Geometry: see drawing. Coordinates: mm, zero at the bounding-box minimum. A direction names the side the tool comes from. Round coordinates to 2 decimals unless told otherwise and drop trailing zeros. Loops run counter-clockwise (first coordinate to the right, second up) from the corner with the lowest first, then second, coordinate; pieces in that order, holes last.
(1) First-contact query: pin 1 Ø1 at (y, z) = (7.5, 36) entering from -X; pin 2 Ø3.5 at (y, z) = (13, 21.8) entering from -X; pin 3 Ø5 at (x, y) = (14, 2) entering from +Z. Flat tips, straight axial feed; report the tip coordinate or a pass-through.
(2) Cut plane C-C, the plane y = 12.25. Output: boundary loops of the cut face in (x, z), and give its area (3 significant figures).
(3) Draft query along Y for the marked faces 1, 2 and 3. Return one class per face: released by +Y, released by -Y, zero draft, split by the parting line, or undercut.
(4) Access query for the marked faces 4 and 5. Directions: +Z, -Z, +X, -X, +Y, -Y. A direction counts if a zero-diameter tool reaches every point of the face in a straight line with its end or side. Return the directions, or none.
(5) Cut plane B-B, the plane x = 21.8. Output: boundary loops of the cut face in (y, z), and give its area (3 significant figures).
(6) Cut plane D-D, the plane x = 33. Output: boundary loops of the cut face in (y, z).
(7) Cut plane A-A, the plane z = 21.8. Output: boundary loops of the cut face in (x, y).
(8) Line query: line 1 (Y direction, x = 29.5, z = 21.8); line 2 (Y direction, x = 42.5, z = 19); line 3 (X direction, y = 6, z = 19). Output: solid intervals per line, ascending.
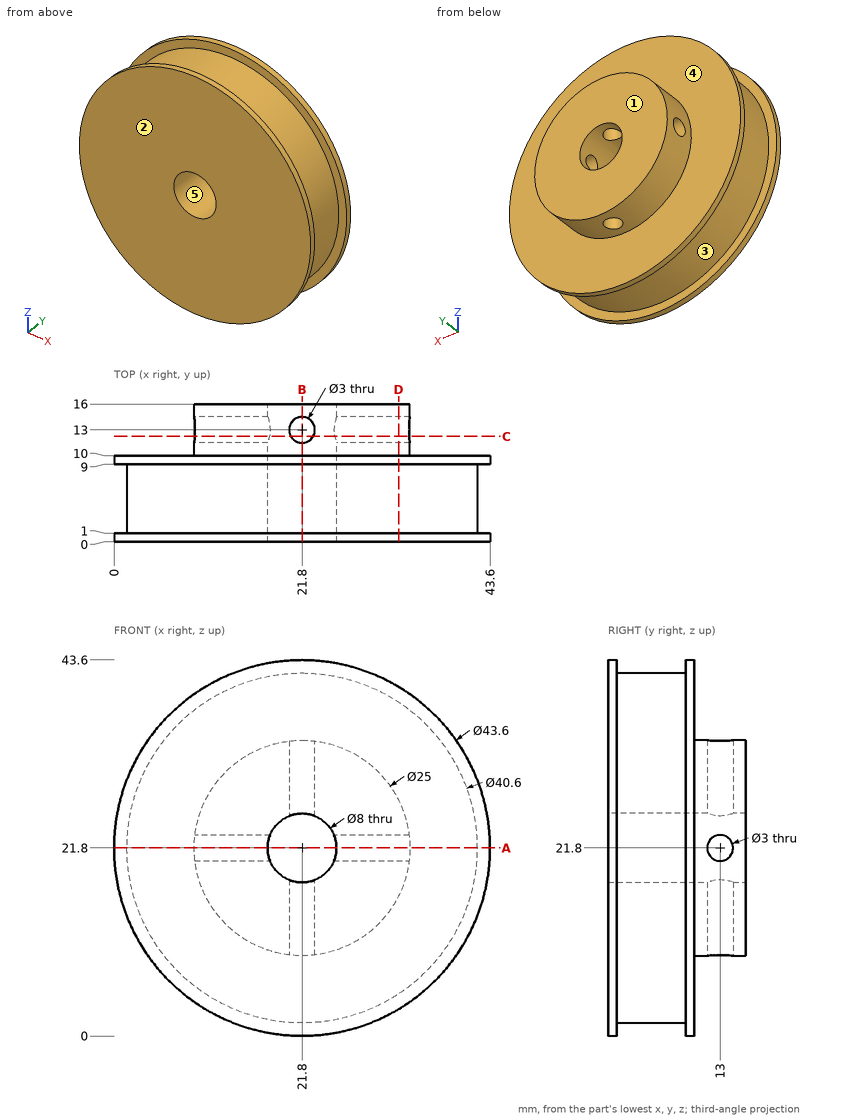
Reported:
1. pin 1: stops at x = 6.82
1. pin 2: stops at x = 9.3
1. pin 3: stops at z = 42.89
2. outline: (9.37, 20.5) arc R12.5 ccw to (20.5, 9.37) - (20.5, 18.02) arc R4 cw to (18.02, 20.5) - close; (9.37, 23.1) - (18.02, 23.1) arc R4 cw to (20.5, 25.58) - (20.5, 34.23) arc R12.5 ccw to start; (23.1, 9.37) arc R12.5 ccw to (34.23, 20.5) - (25.58, 20.5) arc R4 cw to (23.1, 18.02) - close; (23.1, 25.58) arc R4 cw to (25.58, 23.1) - (34.23, 23.1) arc R12.5 ccw to (23.1, 34.23) - close
2. area: 352 mm2
3. face 1: released by +Y
3. face 2: released by -Y
3. face 3: undercut
4. face 4: +Y
4. face 5: +Y, -Y
5. outline: (0, 0) - (1, 0) - (1, 1.5) - (9, 1.5) - (9, 0) - (10, 0) - (10, 9.3) - (11.5, 9.3) - (11.5, 17.8) - (0, 17.8) - close; (0, 25.8) - (11.5, 25.8) - (11.5, 34.3) - (10, 34.3) - (10, 43.6) - (9, 43.6) - (9, 42.1) - (1, 42.1) - (1, 43.6) - (0, 43.6) - close; (14.5, 9.3) - (16, 9.3) - (16, 17.8) - (14.5, 17.8) - close; (14.5, 25.8) - (16, 25.8) - (16, 34.3) - (14.5, 34.3) - close
5. area: 383 mm2
6. outline: (0, 3.1) - (1, 3.1) - (1, 4.87) - (9, 4.87) - (9, 3.1) - (10, 3.1) - (10, 16.25) - (16, 16.25) - (16, 27.35) - (10, 27.35) - (10, 40.5) - (9, 40.5) - (9, 38.73) - (1, 38.73) - (1, 40.5) - (0, 40.5) - close; hole circle Ø3 at (13, 21.8)
7. outline: (0, 0) - (17.8, 0) - (17.8, 11.5) - (9.3, 11.5) - (9.3, 10) - (0, 10) - (0, 9) - (1.5, 9) - (1.5, 1) - (0, 1) - close; (9.3, 14.5) - (17.8, 14.5) - (17.8, 16) - (9.3, 16) - close; (25.8, 0) - (43.6, 0) - (43.6, 1) - (42.1, 1) - (42.1, 9) - (43.6, 9) - (43.6, 10) - (34.3, 10) - (34.3, 11.5) - (25.8, 11.5) - close; (25.8, 14.5) - (34.3, 14.5) - (34.3, 16) - (25.8, 16) - close
8. line 1: y = 0 to 11.5, 14.5 to 16
8. line 2: y = 0 to 1, 9 to 10
8. line 3: x = 1.69 to 18.94, 24.66 to 41.91
